Verification items for the finished model (mm, model axes). A direction names the side the tool comes from. Give positions to 0.01 mm unless a question says otherwise; leave off trailing zeros. Write each loop counter-clockwise with the first axis right and the second up, starting at its lowest first coordinate (ties: lowest second). Pieces come first, ordered by that corner, then holes. Notation, with made-up numbers: (20.25, 16.25) -> (38.25, 16.25) arc R29 cw to (38.25, 53.25) -> close; hole circle Ø5 at (12.25, 23). An arc over 180 degrees is marked (long way). Write item = value, one per line.
from build123d import *

# Parameters (mm, degrees)
SKETCH_1_R          = 10
EXTRUDE_1_DEPTH     = 10
SKETCH_2_W          = 2.284145506
SKETCH_2_H          = 8.27120278
CUT_EXTRUDE_1_DEPTH = 10
CUT_EXTRUDE_2_DEPTH = 2
CUT_EXTRUDE_3_DEPTH = 2
CUT_EXTRUDE_4_DEPTH = 3.5
CUT_EXTRUDE_5_DEPTH = 8
SKETCH_10_R         = 2
CUT_EXTRUDE_6_DEPTH = 1
CUT_EXTRUDE_7_DEPTH = 1
SKETCH_15_R         = 0.598433569
EXTRUDE_5_DEPTH     = 1


with BuildPart() as part:
    # 草圖1 → 填料-伸長1 (new body)
    with BuildSketch(Plane.XY):
        Circle(SKETCH_1_R)
    extrude(amount=EXTRUDE_1_DEPTH)

    # 草圖2 → 除料-伸長1 (cut)
    with BuildSketch(Plane.XY.offset(10)):
        with Locations((-4.477041196, 0.535617876)):
            Rectangle(SKETCH_2_W, SKETCH_2_H)
    extrude(amount=-CUT_EXTRUDE_1_DEPTH, mode=Mode.SUBTRACT)

    # 草圖3 → 除料-伸長2 (cut)
    with BuildSketch(Plane.XY.offset(10)):
        with BuildLine():
            Line((-5.619113949, 4.671219266), (-8.84192912, 4.671219266))
            ThreePointArc((-8.84192912, 4.671219266), (-10.338729016, 0.052381637), (-8.888807861, -4.581385687))
            Line((-8.888807861, -4.581385687), (-5.619113949, -3.599983514))
            Line((-5.619113949, -3.599983514), (-5.619113949, 4.671219266))
        make_face()
    extrude(amount=-CUT_EXTRUDE_2_DEPTH, mode=Mode.SUBTRACT)

    # 草圖4 → 除料-伸長3 (cut)
    with BuildSketch(Plane(origin=(0, 0, 0), x_dir=(-1, 0, 0), z_dir=(0, 0, -1))):
        with BuildLine():
            Line((5.619113949, 4.671219266), (8.84192912, 4.671219266))
            ThreePointArc((8.84192912, 4.671219266), (10.34374886, 0.021931836), (8.86165829, -4.633682375))
            Line((8.86165829, -4.633682375), (5.619113949, -4.633682375))
            Line((5.619113949, -4.633682375), (5.619113949, 4.671219266))
        make_face()
    extrude(amount=-CUT_EXTRUDE_3_DEPTH, mode=Mode.SUBTRACT)

    # 草圖7 → 除料-伸長4 (cut)
    with BuildSketch(Plane.ZY.offset(12.334968443)):
        Polygon((2, 4.671219266), (8, 4.671219266), (8, -4.581385687), (2, -4.633682375), align=None)
    extrude(amount=-CUT_EXTRUDE_4_DEPTH, mode=Mode.SUBTRACT)

    # 草圖9 → 除料-伸長5 (cut)
    with BuildSketch(Plane.XY.offset(8)):
        Polygon((-5.619113949, 4.614635236), (-5.619113949, -3.599983514), (-6.458251574, -3.851851582), (-6.458251574, 4.614635236), align=None)
    extrude(amount=-CUT_EXTRUDE_5_DEPTH, mode=Mode.SUBTRACT)

    # 草圖10 → 除料-伸長6 (cut)
    with BuildSketch(Plane(origin=(1.147174702, 0, 0), x_dir=(-1, 0, 0), z_dir=(0, 0, -1))):
        with Locations((-4.77940273, 2.844632537)):
            Circle(SKETCH_10_R)
    extrude(amount=-CUT_EXTRUDE_6_DEPTH, mode=Mode.SUBTRACT)

    # 草圖11 → 除料-伸長7 (cut)
    with BuildSketch(Plane(origin=(3.950612042, 2.062182751, 0), x_dir=(-1, 0, 0), z_dir=(0, 0, -1))):
        with BuildLine():
            ThreePointArc((-6.134639705, -3.27946709), (-2.337132754, -6.258197714), (2.486199078, -6.08683493))
            ThreePointArc((2.486199078, -6.08683493), (2.754295623, -5.577783265), (2.245243957, -5.30968672))
            ThreePointArc((2.245243957, -5.30968672), (-2.14989891, -5.730336765), (-5.555178734, -2.919945938))
            ThreePointArc((-5.555178734, -2.919945938), (-6.024669795, -2.809976029), (-6.134639705, -3.27946709))
        make_face()
    extrude(amount=-CUT_EXTRUDE_7_DEPTH, mode=Mode.SUBTRACT)

    # 草圖15 → 填料-伸長5 (add)
    with BuildSketch(Plane(origin=(0.571990358, 0, 1), x_dir=(-1, 0, 0), z_dir=(0, 0, -1))):
        with Locations((-5.926577433, 2.844632537)):
            Circle(SKETCH_15_R)
    extrude(amount=EXTRUDE_5_DEPTH)


solid = part.part
Item 1: Material ranges on line 1 (X direction, y = -0.75, z = 5.5); line 2 (Y direction, x = -4.75, z = 9.75); line 3 (Z direction, x = -7.5, y = -1), recorded low to high.
Response values:
line_1 = -8.83 to -6.46, -3.33 to 9.97
line_2 = -8.8 to -3.6, 4.67 to 8.8
line_3 = 2 to 8
Item 2: Go/stop test with flat-tipped pins: P1, Ø0.5, axis at y = -4, z = 1.5, coming from the -X side; P2, Ø2.5, axis at x = -4.5, z = 4, coming from the +Y side; P3, Ø1, axis at x = -7.5, y = -2, coming from the -Z side. Record where each tip stops, or that it passes through.
Response values:
P1 = -5.62
P2 = 9.46
P3 = 2
Item 3: Sectioned sample at A-A on y = 0. Record the cut outline in (x, z).
Response values:
outline = (-8.83, 2) -> (-6.46, 2) -> (-6.46, 8) -> (-8.83, 8) -> close; (-3.33, 0) -> (10, 0) -> (10, 10) -> (-3.33, 10) -> close
Item 4: Sectioned sample at C-C on x = 8.25. Record the cut outline in (y, z).
Response values:
outline = (-5.65, 0) -> (-3.19, 0) -> (-3.19, 1) -> (-2.46, 1) -> (-2.46, 0) -> (5.65, 0) -> (5.65, 10) -> (-5.65, 10) -> close
Item 5: Set-up check for faces 1 (the flat face through (-8, 0, 2)), 2 (the flat face through (3, 0, 0)), 3 (the flat face through (6, -4, 1)), 4 (the flat face through (-8, 0, 8)), 5 (the flat face through (-6, 4.615, 5)): record each of +Z, -Z, +X, -X, +Y, -Y from which the full face is reachable in a straight line by a thin tool's end or side.
Response values:
face_1 = -Z, -X
face_2 = -Z, +X, -X, +Y, -Y
face_3 = -Z
face_4 = +Z, -X
face_5 = +Z, -Z
Item 6: Sectioned sample at D-D on z = 9.75. Record the cut outline in (x, y).
Response values:
outline = (-8.89, -4.58) arc R10 ccw (long way) to (-8.84, 4.67) -> (-3.33, 4.67) -> (-3.33, -3.6) -> (-5.62, -3.6) -> close
Item 7: Mould release check, pull along Y, two halves, no side actions. Record for faces 6 (the flat face through (-4, -3.6, 5)), 7 (the cylindrical face through (10, 0, 5)), 8 (the flat face through (-6.458, 0, 5)): +Y half, -Y half, draft (parallel to the pull), parting line (faces both ways), or undercut.
Response values:
face_6 = undercut
face_7 = parting line
face_8 = undercut
